Geometry check sheet. Reference: the model listing, model coordinates, mm. A direction names the side the tool comes from. Give positions to 0.01 mm unless a question says otherwise; leave off trailing zeros. Loops run counter-clockwise (first coordinate to the right, second up) from the corner with the lowest first, then second, coordinate; pieces in that order, holes last.
1. Tool access check on faces 5 (the flat face through (13, 2.04, 6)), 6 (the flat face through (13, 18.28, 6)), 7 (the cylindrical face through (6.1, 17.8, 5.7)). Record the directions out of +Z, -Z, +X, -X, +Y, -Y that give a thin tool (end or side, any length) a straight path to the whole face; none if there is none.
2. Cross-section at A-A, the plane z = 6. Record the cut outline in (x, y), plus the area to 3 significant figures.
3. Release check for a two-part mould opening along X. For faces 1 (the cylindrical face through (2.103, 18.465, 0.715)), 2 (the cylindrical face through (8.57, 2.55, 5.74)), 3 (the flat face through (13, 10, 1.45)), 4 (the cylindrical face through (20.57, 17.77, 5.74)) record: +X half, -X half, draft (parallel to the pull), parting line (faces both ways), or undercut.
4. Cross-section at B-B, the plane x = 2.54. Record the cut outline in (y, z).
5. Go/stop test with flat-tipped pins: pin 1 Ø1.3 at (x, y) = (24.13, 17.78) entering from -Z; pin 2 Ø4.5 at (x, z) = (15, 7) entering from -Y; pin 3 Ø5 at (x, y) = (16.5, 13) entering from +Z; pin 4 Ø3 at (x, z) = (8.5, 3.5) entering from +Y. Record where each tip stops, or that it passes through.
6. Cross-section at C-C, the plane y = 17.78. Record the cut outline in (x, z), plus the area to 3 significant figures.
7. Cross-section at D-D, the plane x = 10. Record the cut outline in (y, z).
8. Material ranges on L1, parallel to Y at x = 2.54, z = 1; L2, parallel to Y at x = 9.75, z = 7.5; L3, parallel to Z at x = 8.25, y = 12.25, recorded low to high.
from build123d import *

# Parameters (mm, degrees)
F0_W     = 26.67
F0_H     = 20.32
F1_DEPTH = 1.45
F3_D     = 1.6256
F5_DEPTH = 8.7
F6_DEPTH = 2.1


with BuildPart() as f1:
    # F0 (on Top) → F1 (new body)
    with BuildSketch(Plane.XY):
        with Locations((13.335, 10.16)):
            Rectangle(F0_W, F0_H)
    extrude(amount=F1_DEPTH)

    # F3 (through all)
    with Locations(Plane.XY.offset(1.45)):
        with Locations((2.54, 17.78), (2.54, 2.54), (24.13, 2.54), (24.13, 17.78)):
            Hole(F3_D / 2)

    # F4 (on face) → F5 (join)
    with BuildSketch(Plane.XY.offset(1.45)):
        with BuildLine():
            Line((20.07, 18.28), (6.6, 18.28))
            ThreePointArc((6.6, 18.28), (6.1, 17.78), (6.6, 17.28))
            Line((6.6, 17.28), (20.07, 17.28))
            ThreePointArc((20.07, 17.28), (20.57, 17.78), (20.07, 18.28))
        make_face()
        with BuildLine():
            Line((17.6, 3.04), (9.07, 3.04))
            ThreePointArc((9.07, 3.04), (8.57, 2.54), (9.07, 2.04))
            Line((9.07, 2.04), (17.6, 2.04))
            ThreePointArc((17.6, 2.04), (18.1, 2.54), (17.6, 3.04))
        make_face()
    extrude(amount=F5_DEPTH)

    # F4 (on face) → F6 (join)
    with BuildSketch(Plane.XY.offset(1.45)):
        with BuildLine():
            Line((20.07, 18.28), (6.6, 18.28))
            ThreePointArc((6.6, 18.28), (6.1, 17.78), (6.6, 17.28))
            Line((6.6, 17.28), (20.07, 17.28))
            ThreePointArc((20.07, 17.28), (20.57, 17.78), (20.07, 18.28))
        make_face()
        with BuildLine():
            Line((17.6, 3.04), (9.07, 3.04))
            ThreePointArc((9.07, 3.04), (8.57, 2.54), (9.07, 2.04))
            Line((9.07, 2.04), (17.6, 2.04))
            ThreePointArc((17.6, 2.04), (18.1, 2.54), (17.6, 3.04))
        make_face()
    extrude(amount=-F6_DEPTH)


solid = f1.part
Result:
1. face 5: +Z, +X, -X, -Y
1. face 6: +Z, +X, -X, +Y
1. face 7: +Z, -X
2. outline: (6.6, 17.28) - (20.07, 17.28) arc R0.5 ccw to (20.07, 18.28) - (6.6, 18.28) arc R0.5 ccw to start; (9.07, 2.04) - (17.6, 2.04) arc R0.5 ccw to (17.6, 3.04) - (9.07, 3.04) arc R0.5 ccw to start
2. area: 23.6 mm2
3. face 1: undercut
3. face 2: -X half
3. face 3: draft
3. face 4: +X half
4. outline: (0, 0) - (1.73, 0) - (1.73, 1.45) - (0, 1.45) - close; (3.35, 0) - (16.97, 0) - (16.97, 1.45) - (3.35, 1.45) - close; (18.59, 0) - (20.32, 0) - (20.32, 1.45) - (18.59, 1.45) - close
5. pin 1: passes through
5. pin 2: stops at y = 2.04
5. pin 3: stops at z = 1.45
5. pin 4: stops at y = 18.28
6. outline: (0, 0) - (1.73, 0) - (1.73, 1.45) - (0, 1.45) - close; (3.35, 0) - (6.1, 0) - (6.1, -0.65) - (20.57, -0.65) - (20.57, 0) - (23.32, 0) - (23.32, 1.45) - (20.57, 1.45) - (20.57, 10.15) - (6.1, 10.15) - (6.1, 1.45) - (3.35, 1.45) - close; (24.94, 0) - (26.67, 0) - (26.67, 1.45) - (24.94, 1.45) - close
6. area: 169 mm2
7. outline: (0, 0) - (2.04, 0) - (2.04, -0.65) - (3.04, -0.65) - (3.04, 0) - (17.28, 0) - (17.28, -0.65) - (18.28, -0.65) - (18.28, 0) - (20.32, 0) - (20.32, 1.45) - (18.28, 1.45) - (18.28, 10.15) - (17.28, 10.15) - (17.28, 1.45) - (3.04, 1.45) - (3.04, 10.15) - (2.04, 10.15) - (2.04, 1.45) - (0, 1.45) - close
8. L1: y = 0 to 1.73, 3.35 to 16.97, 18.59 to 20.32
8. L2: y = 2.04 to 3.04, 17.28 to 18.28
8. L3: z = 0 to 1.45
